Can you work these out from the model? Positions are in its coordinate system, mm. Coordinates: 2 decimals unless noted, no trailing zeros. Order: outer loops, then holes, each group sorted by start corner. A loop starts at its lowest first (then second) coordinate and runs counter-clockwise, first axis right, second up.
```python
from build123d import *

# Parameters (mm, degrees)
SKETCH_1_W         = 24
SKETCH_1_H         = 24
SKETCH_1_W_2       = 20
SKETCH_1_H_2       = 20
EXTRUDE_1_DEPTH    = 271
HOLE_WIZARD_M3_3_D = 2.5


with BuildPart() as part:
    # 草图1 → 凸台-拉伸1 (new, symmetric)
    with BuildSketch(Plane.XY):
        Rectangle(SKETCH_1_W, SKETCH_1_H)
        Rectangle(SKETCH_1_W_2, SKETCH_1_H_2, mode=Mode.SUBTRACT)
    extrude(amount=EXTRUDE_1_DEPTH, both=True)

    # M3 螺纹孔的螺纹孔钻头3 (through all)
    with Locations(Plane(origin=(-12, 0, -135), x_dir=(0, -1, 0), z_dir=(-1, 0, 0))):
        with Locations((0, 0)):
            hole_wizard_m3_3 = Hole(HOLE_WIZARD_M3_3_D / 2)

    # 镜向1: M3 螺纹孔的螺纹孔钻头3 across plane
    add(hole_wizard_m3_3.mirror(Plane.XY), mode=Mode.SUBTRACT)


solid = part.part
```
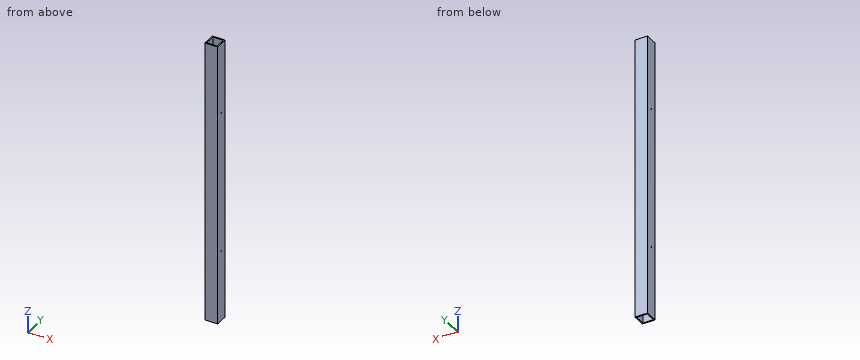
1. Please list where these lines run through material, in increasing order: probe 1 along Z at (x, y) = (10.65, 0); probe 2 along Y at (x, z) = (-0.75, -226); probe 3 along Y at (x, z) = (10.9, 135).
Completed:
probe 1: z = -271 to -136.25, -133.75 to 133.75, 136.25 to 271
probe 2: y = -12 to -10, 10 to 12
probe 3: y = -12 to -1.25, 1.25 to 12
2. Imagine slicing it at C-C on z = 23.5. Please give me the cut outline in (x, y), then the cut area to 3 significant figures.
Completed:
outline: (-12, -12) - (12, -12) - (12, 12) - (-12, 12) - close; hole (-10, -10) - (10, -10) - (10, 10) - (-10, 10) - close
area: 176 mm2
3. Imagine slicing it at A-A on y = -5. Please give me the cut outline in (x, z), then the cut area to 3 significant figures.
Completed:
outline: (-12, -271) - (-10, -271) - (-10, 271) - (-12, 271) - close; (10, -271) - (12, -271) - (12, 271) - (10, 271) - close
area: 2,170 mm2
4. I'm going to push a flat-ended pin straight in: pin 1 (1.5 mm diameter, centred on y = 0, z = -135, fed in from -X). Where does the tip first touch, or does it pass through?
Completed:
pin 1: passes through
